from build123d import *

# Parameters (mm, degrees)
F1_DEPTH = 15
F3_DEPTH = 15


with BuildPart() as f1:
    # F0 (on Top) → F1 (new body)
    with BuildSketch(Plane.XY):
        Polygon((0, -120), (0, 0), (-120, 0), (-120, -60), (-60, -60), (-60, -120), align=None)
    extrude(amount=F1_DEPTH)

    # F2 (on Front) → F3 (join)
    with BuildSketch(Plane.XZ):
        Polygon((-120, 0), (0, 0), (0, 45), (-40, 45), (-40, 65), (-80, 65), (-80, 45), (-120, 45), align=None)
    extrude(amount=F3_DEPTH)


solid = f1.part
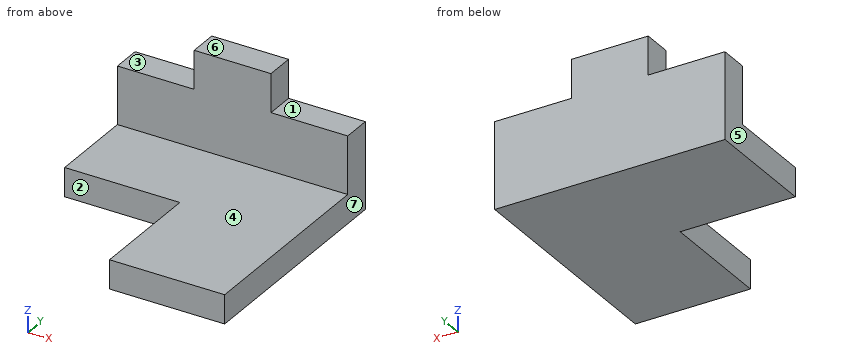
Verification items for the finished model (mm, model axes). Face numbers are marked on the shaded views. A direction names the side the tool comes from. Round coordinates to 2 decimals unless told otherwise and drop trailing zeros. Write each loop counter-clockwise with the first axis right and the second up, starting at its lowest first coordinate (ties: lowest second). Pieces come first, ordered by that corner, then holes.
(1) Depth check by flat-ended pin: pin 1 Ø3 at (x, z) = (-68, 58.5) entering from +Y; pin 2 Ø7.5 at (x, z) = (-95, 11) entering from -Y; pin 3 Ø7.5 at (y, z) = (-91.5, 8) entering from -X; pin 4 Ø7.5 at (y, z) = (-8, 54) entering from +X. Enter the tip coordinate at first touch or a pass-through.
Returned:
pin 1: stops at y = 0
pin 2: stops at y = -60
pin 3: stops at x = -60
pin 4: stops at x = -40
(2) Section check D-D (z = 52). Enter the section's corners in (x, y).
Returned:
outline: (-80, -15) - (-40, -15) - (-40, 0) - (-80, 0) - close
(3) Section check A-A (y = -13). Enter the section's corners in (x, z).
Returned:
outline: (-120, 0) - (0, 0) - (0, 45) - (-40, 45) - (-40, 65) - (-80, 65) - (-80, 45) - (-120, 45) - close
(4) Section check B-B (x = -13). Enter the section's corners in (y, z), plus the area to 3 significant figures.
Returned:
outline: (-120, 0) - (0, 0) - (0, 45) - (-15, 45) - (-15, 15) - (-120, 15) - close
area: 2,250 mm2
(5) Mould release check, pull along X, two halves, no side actions. Record for the marked faces 5, 6 and 7: pulls with the +X half, pulls with the -X half, needs draft (parallel to the pull), parting line crosses it, or undercut.
Returned:
face 5: pulls with the -X half
face 6: needs draft
face 7: pulls with the +X half
(6) Access from +Z, -Z, +X, -X, +Y, -Y to the whole of each face (thin tool, end or side, straight path). Record for the marked faces 1, 2, 3 and 4.
Returned:
face 1: +Z, +X, +Y, -Y
face 2: +Z, -Z, -X, -Y
face 3: +Z, -X, +Y, -Y
face 4: +Z, +X, -X, -Y
(7) Section check C-C (x = -58.5). Enter the section's corners in (y, z).
Returned:
outline: (-120, 0) - (0, 0) - (0, 65) - (-15, 65) - (-15, 15) - (-120, 15) - close
(8) Material ranges on line 1 (Z direction, x = -29, y = -48.5); line 2 (X direction, y = -83, z = 13.5); line 3 (Y direction, x = -112, z = 29), recorded low to high.
Returned:
line 1: z = 0 to 15
line 2: x = -60 to 0
line 3: y = -15 to 0
